Design review of the part built by this model. Coordinates are the model's own, in mm. A direction names the side the tool comes from. Coordinates: 2 decimals unless noted, no trailing zeros. Write each loop counter-clockwise with the first axis right and the second up, starting at its lowest first coordinate (ties: lowest second). Pieces come first, ordered by that corner, then holes. Notation, with made-up numbers: (-32.75, 16) - (-27.75, 16) arc R19 cw to (-27.75, 28) - close; hole circle Ø1 at (71.25, -31.75). An arc over 180 degrees is marked (long way). Answer as CSV lines item,"result". Start each with the question number.
Q1. Clearance check with flat-ended pins moving along their axes: pin 1 (4.5 mm diameter, centred on x = -7.75, z = 7.75, fed in from +Y); pin 2 (4.5 mm diameter, centred on x = 7.75, z = 7.75, fed in from -Y); pin 3 (1.2 mm diameter, centred on y = 2, z = -0.5, fed in from +X); pin 4 (1.2 mm diameter, centred on x = -0.5, y = 2, fed in from +Z). State where each tip first meets the part, or that it passes through.
Q2. Machinability: for faces 1 (the face through (0, 0, 3)), 2 (the face through (-0.49, 0.25, -2.21)), 3 (the face through (0, 2, 1.9)), which of the approach directions +Z, -Z, +X, -X, +Y, -Y give a long, thin tool a straight path to every point of the face, cutting with its end or side? Answer none if there is none.
Q3. We need section C-C (x = -6.5). Write out the cut boundary in (y, z).
Q4. We need section D-D (z = 0). Write out the cut boundary in (x, y).
Q5. Mouldability with a two-part tool opening along Z and no side actions: class faces 4 (the face through (0, 0.5, 0)), 5 (the face through (2.45, 2, 0)), 6 (the face through (10.109, 0.493, 10.047)) as pulls with the +Z half, pulls with the -Z half, needs draft (parallel to the pull), parting line crosses it, or undercut.
Q6. For line 1 along Z through (x, y) = (7.75, 0.55); line 2 along X through (y, z) = (0.55, -9), list the stretches that pass through material, from the lowest coordinate up. Write a range as [from, to].
Q7. We need section B-B (x = 0). Write out the cut boundary in (y, z), plus the area to 3 significant figures.
Q8. We need section A-A (z = 7.75). Write out the cut boundary in (x, y).
Autodesk Inventor part; units mm, degrees
ref_plane "YZ Plane" through (0, 0, 0) normal (1, 0, 0) x (0, 1, 0)
ref_plane "XZ Plane" through (0, 0, 0) normal (0, 1, 0) x (-1, 0, 0)
ref_plane "XY Plane" through (0, 0, 0) normal (0, 0, 1) x (1, 0, 0)
sketch "Skizze1" plane through (0, 0, 0) normal (0, 1, 0) x (-1, 0, 0)
  line L0 (7.25, -11.25) -> (-7.25, -11.25)
  line L1 (-11.25, -7.25) -> (-11.25, 7.25)
  line L2 (-7.25, 11.25) -> (7.25, 11.25)
  line L3 (11.25, 7.25) -> (11.25, -7.25)
  line L4 (11.25, -11.25) -> (-11.25, 11.25) construction
  line L5 (-11.25, -11.25) -> (11.25, 11.25) construction
  arc A0 (-7.25, 11.25) -> (-11.25, 7.25) centre (-7.25, 7.25) ccw
  arc A1 (11.25, 7.25) -> (7.25, 11.25) centre (7.25, 7.25) ccw
  arc A2 (7.25, -11.25) -> (11.25, -7.25) centre (7.25, -7.25) ccw
  arc A3 (-11.25, -7.25) -> (-7.25, -11.25) centre (-7.25, -7.25) ccw
  point P0 (0, 0)
  dimension "d0" = 22.5
  dimension "d1" = 22.5
  dimension "d2" = 4
extrude "Extrusion1" add sketch "Skizze1" along normal blind 1
sketch "Skizze2" plane through (0, 1, 0) normal (0, 1, 0) x (1, 0, 0)
  line L0 (-7.25, -11.25) -> (7.25, -11.25)
  arc A0 (7.25, -11.25) -> (11.25, -7.25) centre (7.25, -7.25) ccw
  line L1 (11.25, -7.25) -> (11.25, 7.25)
  arc A1 (11.25, 7.25) -> (7.25, 11.25) centre (7.25, 7.25) ccw
  line L2 (7.25, 11.25) -> (-7.25, 11.25)
  arc A2 (-7.25, 11.25) -> (-11.25, 7.25) centre (-7.25, 7.25) ccw
  line L3 (-11.25, 7.25) -> (-11.25, -7.25)
  arc A3 (-11.25, -7.25) -> (-7.25, -11.25) centre (-7.25, -7.25) ccw
  line L4 (2.45, -1.9) -> (-2.45, -1.9)
  line L5 (-2.45, -1.9) -> (-2.45, 1.9)
  line L6 (-2.45, 1.9) -> (2.45, 1.9)
  line L7 (2.45, 1.9) -> (2.45, -1.9)
  line L8 (2.45, -1.9) -> (-2.45, 1.9) construction
  line L9 (-2.45, -1.9) -> (2.45, 1.9) construction
  point P0 (0, 0)
  dimension "d5" = 4.9
  dimension "d6" = 3.8
extrude "Extrusion2" add sketch "Skizze2" along normal blind 1.5 contours L4 L5 L6 L7
sketch "Skizze3" plane through (0, 1, 0) normal (0, 1, 0) x (1, 0, 0)
  line L0 (2.45, 1.9) -> (2.45, -1.9)
  line L1 (2.45, -1.9) -> (-2.45, -1.9)
  line L2 (-2.45, -1.9) -> (-2.45, 1.9)
  line L3 (-2.45, 1.9) -> (2.45, 1.9)
  line L4 (-7.25, -11.25) -> (7.25, -11.25)
  arc A0 (7.25, -11.25) -> (11.25, -7.25) centre (7.25, -7.25) ccw
  line L5 (11.25, -7.25) -> (11.25, 7.25)
  arc A1 (11.25, 7.25) -> (7.25, 11.25) centre (7.25, 7.25) ccw
  line L6 (7.25, 11.25) -> (-7.25, 11.25)
  arc A2 (-7.25, 11.25) -> (-11.25, 7.25) centre (-7.25, 7.25) ccw
  line L7 (-11.25, 7.25) -> (-11.25, -7.25)
  arc A3 (-11.25, -7.25) -> (-7.25, -11.25) centre (-7.25, -7.25) ccw
  line L8 (-7.75, 7.75) -> (7.75, 7.75) construction
  line L9 (7.75, 7.75) -> (7.75, -7.75) construction
  line L10 (7.75, -7.75) -> (-7.75, -7.75) construction
  line L11 (-7.75, -7.75) -> (-7.75, 7.75) construction
  line L12 (-7.75, 7.75) -> (7.75, -7.75) construction
  line L13 (7.75, 7.75) -> (-7.75, -7.75) construction
  point P0 (0, 0)
  dimension "d9" = 15.5
  dimension "d10" = 15.5
hole "Bohrung1" at (7.75, 1, 7.75) at (-7.75, 1, 7.75) at (-7.75, 1, -7.75) at (7.75, 1, -7.75) direction (0, -1, 0) diameter 4 depth 3 tip angle 118
sketch "Skizze4" plane through (0, 0, 0) normal (0, -1, 0) x (1, 0, 0)
  circle A0 centre (0, 0) radius 2.2643
extrude "Extrusion3" cut sketch "Skizze4" against normal blind 0.5
properties part number "00_AS5600_rotational_encoder_i2c"
Results list:
1,pin 1,"stops at y = 1"
1,pin 2,"stops at y = 0"
1,pin 3,"stops at x = 2.45"
1,pin 4,"stops at z = 1.9"
2,face 1,"+Z, -Z, +X, -X, -Y"
2,face 2,"-Y"
2,face 3,"+Z, +X, -X, +Y"
3,outline,"(0, -11.25) - (1, -11.25) - (1, -9.31) - (0, -9.31) - close; (0, -6.19) - (1, -6.19) - (1, 6.19) - (0, 6.19) - close; (0, 9.31) - (1, 9.31) - (1, 11.25) - (0, 11.25) - close"
4,outline,"(-11.25, 0) - (-2.26, 0) - (-2.26, 0.5) - (2.26, 0.5) - (2.26, 0) - (11.25, 0) - (11.25, 1) - (2.45, 1) - (2.45, 2.5) - (-2.45, 2.5) - (-2.45, 1) - (-11.25, 1) - close"
5,face 4,"undercut"
5,face 5,"needs draft"
5,face 6,"pulls with the +Z half"
6,line 1,"z = [-11.22, -9.75], [-5.75, 5.75], [9.75, 11.22]"
6,line 2,"x = [-10.85, -9.31], [-6.19, 6.19], [9.31, 10.85]"
7,outline,"(0, -11.25) - (1, -11.25) - (1, -1.9) - (2.5, -1.9) - (2.5, 1.9) - (1, 1.9) - (1, 11.25) - (0, 11.25) - (0, 2.26) - (0.5, 2.26) - (0.5, -2.26) - (0, -2.26) - close"
7,area,"25.9 mm2"
8,outline,"(-11.22, 0) - (-9.75, 0) - (-9.75, 1) - (-11.22, 1) - close; (-5.75, 0) - (5.75, 0) - (5.75, 1) - (-5.75, 1) - close; (9.75, 0) - (11.22, 0) - (11.22, 1) - (9.75, 1) - close"
